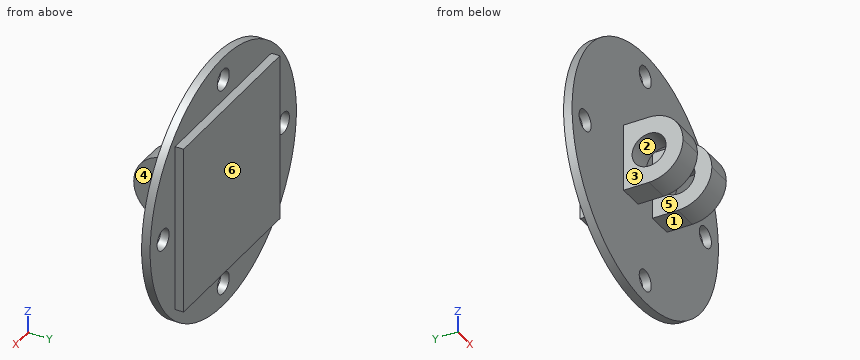
from build123d import *

# Parameters (mm, degrees)
SKETCH1_R           = 76
BOSS_EXTRUDE1_DEPTH = 5
SKETCH1_5_R         = 6.25
CUT_EXTRUDE2_DEPTH  = 5
SKETCH2_W           = 100
SKETCH2_H           = 100
BOSS_EXTRUDE2_DEPTH = 5
SKETCH3_W           = 15
SKETCH3_H           = 40
BOSS_EXTRUDE3_DEPTH = 35
FILLET3_R           = 20
SKETCH5_R           = 10
CUT_EXTRUDE3_DEPTH  = 72


with BuildPart() as part:
    # Sketch1 → Boss-Extrude1 (new body)
    with BuildSketch(Plane(origin=(0, 0, 0), x_dir=(1, 0, 0), z_dir=(0, 1, 0))):
        with Locations(Location((0, 0, 0), (0, 0, 270))):
            Circle(SKETCH1_R)
    extrude(amount=BOSS_EXTRUDE1_DEPTH)

    # Sketch1<5> → Cut-Extrude2 (cut)
    with BuildSketch(Plane(origin=(0, 0, 0), x_dir=(1, 0, 0), z_dir=(0, 1, 0))):
        with Locations(Location((-62.5, 0, 0), (0, 0, 270))):
            Circle(SKETCH1_5_R)
        with Locations(Location((0, 62.5, 0), (0, 0, 270))):
            Circle(SKETCH1_5_R)
        with Locations(Location((62.5, 0, 0), (0, 0, 270))):
            Circle(SKETCH1_5_R)
        with Locations(Location((0, -62.5, 0), (0, 0, 270))):
            Circle(SKETCH1_5_R)
    extrude(amount=CUT_EXTRUDE2_DEPTH, mode=Mode.SUBTRACT)

    # Sketch2 → Boss-Extrude2 (add)
    with BuildSketch(Plane(origin=(0, 5, 0), x_dir=(1, 0, 0), z_dir=(0, 1, 0))):
        Rectangle(SKETCH2_W, SKETCH2_H)
    extrude(amount=BOSS_EXTRUDE2_DEPTH)

    # Sketch3 → Boss-Extrude3 (add)
    with BuildSketch(Plane.XZ):
        with Locations((-15, 0)):
            Rectangle(SKETCH3_W, SKETCH3_H)
        with Locations((15, 0)):
            Rectangle(SKETCH3_W, SKETCH3_H)
    extrude(amount=BOSS_EXTRUDE3_DEPTH)

    # Fillet3
    fillet3_edges = [part.edges().sort_by_distance(p)[0] for p in [
        (15, -35, -20),
        (15, -35, 20),
        (-15, -35, 20),
        (-15, -35, -20),
    ]]
    fillet(fillet3_edges, radius=FILLET3_R - 0.0001)  # a hair under: the kernel refuses the full size

    # Sketch5 → Cut-Extrude3 (cut)
    with BuildSketch(Plane(origin=(22.5, 0, 0), x_dir=(0, 0, -1), z_dir=(1, 0, 0))):
        with Locations((0, -15)):
            Circle(SKETCH5_R)
    extrude(amount=-CUT_EXTRUDE3_DEPTH, mode=Mode.SUBTRACT)


solid = part.part
Check sheet for the modelled part. Datum: model origin and axes. Units: mm. Face numbers are marked on the shaded views. A direction names the side the tool comes from. Give positions to 0.01 mm unless a question says otherwise; leave off trailing zeros. Write each loop counter-clockwise with the first axis right and the second up, starting at its lowest first coordinate (ties: lowest second). Pieces come first, ordered by that corner, then holes. Notation, with made-up numbers: (-7.75, 49) -> (18.25, 49) arc R8 cw to (18.25, 57) -> close; hole circle Ø9 at (37.5, 85.25). An arc over 180 degrees is marked (long way). Write item = value, one per line.
Item 1: Release check for a two-part mould opening along X. For the marked faces 4, 5 and 6 record: +X half, -X half, draft (parallel to the pull), parting line (faces both ways), or undercut.
Output:
face_4 = +X half
face_5 = undercut
face_6 = draft
Item 2: Sectioned sample at B-B on z = -2.5. Count the separate pieces of the cut face and the enclosed holes in it, and give its area (3 significant figures).
Output:
separate_pieces = 5
enclosed_holes = 0
area = 1,610 mm^2
Item 3: Tool access check on the marked faces 1, 2 and 3. Record the directions out of +Z, -Z, +X, -X, +Y, -Y that give a thin tool (end or side, any length) a straight path to the whole face; none if there is none.
Output:
face_1 = -Z, +X, -X, -Y
face_2 = +X, -X
face_3 = +Z, -Z, -X, -Y
Item 4: Sectioned sample at C-C on y = -31. Record the boundary of the cut face in (x, z).
Output:
outline = (-22.5, -12) -> (-7.5, -12) -> (-7.5, 12) -> (-22.5, 12) -> close; (7.5, -12) -> (22.5, -12) -> (22.5, 12) -> (7.5, 12) -> close
Item 5: Sectioned sample at A-A on x = 0. Record the boundary of the cut face in (y, z), and give its area (4 significant figures).
Output:
outline = (0, -76) -> (5, -76) -> (5, -68.75) -> (0, -68.75) -> close; (0, -56.25) -> (5, -56.25) -> (5, -50) -> (10, -50) -> (10, 50) -> (5, 50) -> (5, 56.25) -> (0, 56.25) -> close; (0, 68.75) -> (5, 68.75) -> (5, 76) -> (0, 76) -> close
area = 1,135 mm^2
Item 6: Scan lines: probe 1 along Y at (x, z) = (45, -31.5); probe 2 along Y at (x, z) = (-41.5, 55); probe 3 along Y at (x, z) = (16, 4). Record each from-to range of solid material in increasing order. Write a range as from..to.
Output:
probe_1 = 0..10
probe_2 = 0..5
probe_3 = -34.6..-24.17, -5.83..10
Item 7: Gauge pin test, flat ends, axial feed: pin 1 (1.5 mm diameter, centred on x = 2, y = 7, fed in from +Z); pin 2 (10 mm diameter, centred on x = -62.5, z = 0, fed in from +Y); pin 3 (5 mm diameter, centred on y = 5, z = -22, fed in from +X); pin 4 (5.5 mm diameter, centred on y = 7.5, z = -19, fed in from -X). Record the tip position at first contact, or that the pin passes through.
Output:
pin_1 = 50
pin_2 = through
pin_3 = 73.46
pin_4 = -73.87
